Could you check a few things on this drawing? It's one solid part, dimensions in mm from its lowest x, y, z. Give positions to 0.01 mm unless a question says otherwise; leave off trailing zeros. Order: outer loops, then holes, each group sorted by start corner. A loop starts at its lowest first (then second) coordinate and runs counter-clockwise, first axis right, second up. Notation, with made-up numbers: (10, -14.5) -> (61, -14.5) arc R28 ccw to (61, 11.5) -> close; hole circle Ø6 at (38, 13). An arc over 180 degrees is marked (long way). Answer as CSV lines item,"result".
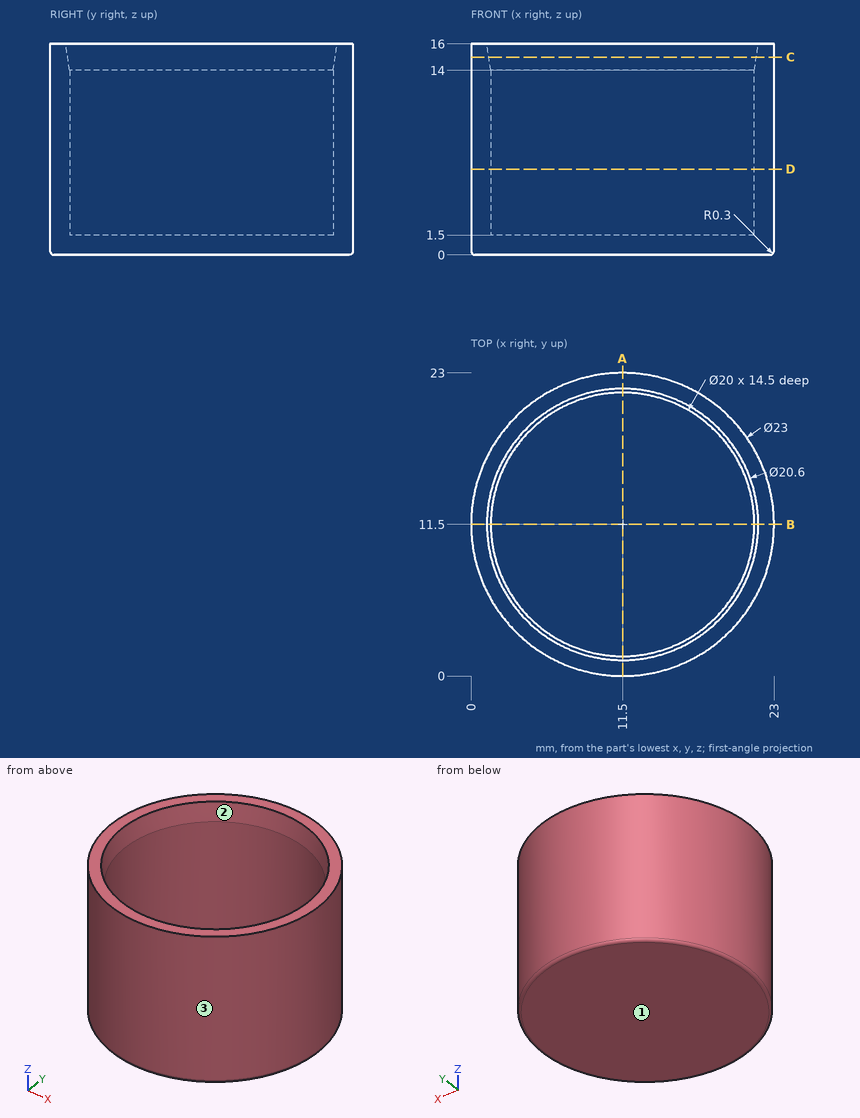
Item 1: Please list where these lines run through material, in increasing order: line 1 along Y through (x, z) = (11.5, 5); line 2 along Z through (x, y) = (18.5, 17.5); line 3 along Y through (x, z) = (9.5, 3).
Numbers:
line 1,"y = 0 to 1.5, 21.5 to 23"
line 2,"z = 0 to 1.5"
line 3,"y = 0.18 to 1.7, 21.3 to 22.82"
Item 2: Imagine slicing it at A-A, the plane x = 11.5. Please give me the cut outline in (y, z).
Numbers:
outline,"(0, 0.3) arc R0.3 ccw to (0.3, 0) -> (22.7, 0) arc R0.3 ccw to (23, 0.3) -> (23, 16) -> (21.8, 16) -> (21.5, 14) -> (21.5, 1.5) -> (1.5, 1.5) -> (1.5, 14) -> (1.2, 16) -> (0, 16) -> close"
Item 3: We'd pull the mould along Y, two halves only. Please class the marked faces 1, 2 and 3: released by +Y, released by -Y, zero draft, split by the parting line, or undercut.
Numbers:
face 1,"zero draft"
face 2,"undercut"
face 3,"split by the parting line"
Item 4: Imagine slicing it at D-D, the plane z = 6.5. Please give me the cut outline in (x, y).
Numbers:
outline,"circle Ø23 at (11.5, 11.5); hole circle Ø20 at (11.5, 11.5)"
Item 5: For pin 1 (3 mm diameter, centred on x = 12.5, y = 14.5, fed in from +Z); pin 2 (1 mm diameter, centred on x = 11.5, y = 9, fed in from -Z); pin 3 (5 mm diameter, centred on x = 2.5, z = 4, fed in from +Y); pin 4 (8 mm diameter, centred on x = 6, z = 4.5, fed in from -Y), each with a flat end and sliding along its axis, tell me the tip position at first contact or that it passes through.
Numbers:
pin 1,"stops at z = 1.5"
pin 2,"stops at z = 0"
pin 3,"stops at y = 20.99"
pin 4,"stops at y = 0.1"
Item 6: Imagine slicing it at C-C, the plane z = 15. Please give me the cut outline in (x, y), then the cut area to 3 significant figures.
Numbers:
outline,"circle Ø23 at (11.5, 11.5); hole circle Ø20.3 at (11.5, 11.5)"
area,"91.8 mm²"
